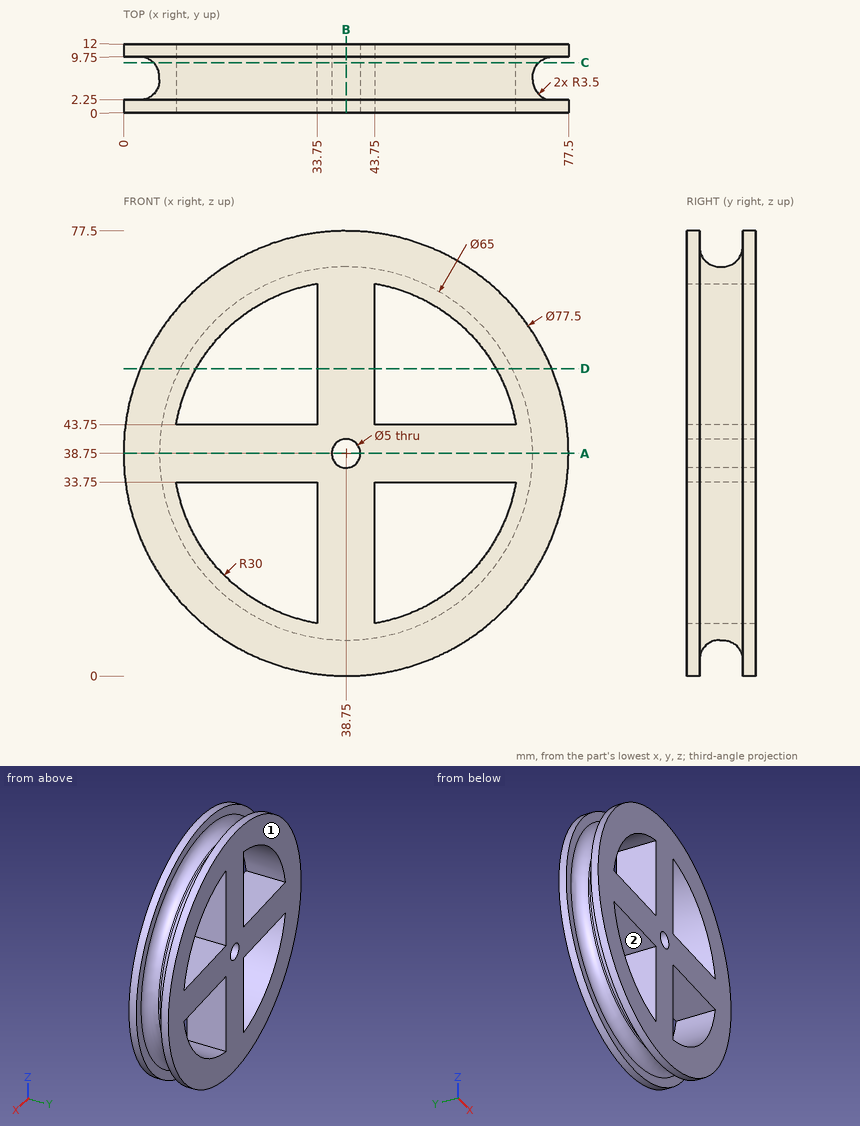
Verification items for this drawing (mm, ordinates from the low corner). A direction names the side the tool comes from. Round coordinates to 2 decimals unless told otherwise and drop trailing zeros. Order: outer loops, then holes, each group sorted by start corner. A loop starts at its lowest first (then second) coordinate and runs counter-clockwise, first axis right, second up. Notation, with made-up numbers: (31, 30.5) - (51, 30.5) arc R16 cw to (51, 60.5) - close; hole circle Ø5 at (64, 35). An arc over 180 degrees is marked (long way). Use CSV: the item, a comma, the result in double quotes.
(1) Section check C-C on y = 8.75. Record the boundary of the cut face in (x, z), and give its area (3 significant figures).
Entries:
outline,"circle Ø67.1 at (38.75, 38.75); hole (9.17, 33.75) arc R30 ccw to (33.75, 9.17) - (33.75, 33.75) - close; hole (9.17, 43.75) - (33.75, 43.75) - (33.75, 68.33) arc R30 ccw to start; hole circle Ø5 at (38.75, 38.75); hole (43.75, 9.17) arc R30 ccw to (68.33, 33.75) - (43.75, 33.75) - close; hole (43.75, 43.75) - (68.33, 43.75) arc R30 ccw to (43.75, 68.33) - close"
area,"1,780 mm^2"
(2) Access from +Z, -Z, +X, -X, +Y, -Y to the whole of each face (thin tool, end or side, straight path). Record for the marked faces 1 and 2.
Entries:
face 1,"+Z, -Z, +X, -X, +Y"
face 2,"+Y, -Y"
(3) Section check A-A on z = 38.75. Record the boundary of the cut face in (x, y).
Entries:
outline,"(0, 0) - (36.25, 0) - (36.25, 12) - (0, 12) - (0, 9.75) - (2.75, 9.75) arc R3.5 cw to (6.25, 6.25) - (6.25, 5.75) arc R3.5 cw to (2.75, 2.25) - (0, 2.25) - close; (41.25, 0) - (77.5, 0) - (77.5, 2.25) - (74.75, 2.25) arc R3.5 cw to (71.25, 5.75) - (71.25, 6.25) arc R3.5 cw to (74.75, 9.75) - (77.5, 9.75) - (77.5, 12) - (41.25, 12) - close"
(4) Section check B-B on x = 38.75. Record the boundary of the cut face in (y, z), and give its area (3 significant figures).
Entries:
outline,"(0, 0) - (2.25, 0) - (2.25, 2.75) arc R3.5 cw to (5.75, 6.25) - (6.25, 6.25) arc R3.5 cw to (9.75, 2.75) - (9.75, 0) - (12, 0) - (12, 36.25) - (0, 36.25) - close; (0, 41.25) - (12, 41.25) - (12, 77.5) - (9.75, 77.5) - (9.75, 74.75) arc R3.5 cw to (6.25, 71.25) - (5.75, 71.25) arc R3.5 cw to (2.25, 74.75) - (2.25, 77.5) - (0, 77.5) - close"
area,"787 mm^2"
(5) Section check D-D on z = 53.5. State how many separate pieces and enclosed holes the cut face has, and give its area (3 significant figures).
Entries:
separate pieces,"3"
enclosed holes,"0"
area,"262 mm^2"
(6) Gauge pin test, flat ends, axial feed: pin 1 Ø8 at (x, z) = (31.5, 8.5) entering from -Y; pin 2 Ø6 at (x, y) = (51.5, 9) entering from -Z; pin 3 Ø3 at (x, z) = (38.75, 38.75) entering from +Y; pin 4 Ø1 at (x, y) = (21.5, 5) entering from +Z. Record the tip position at first contact, or that the pin passes through.
Entries:
pin 1,"y = 0"
pin 2,"z = 1.27"
pin 3,"through"
pin 4,"z = 66.73"
(7) Thickness scan on probe 1 along X at (y, z) = (10.75, 23); probe 2 along X at (y, z) = (7.5, 44); probe 3 along Y at (x, z) = (71, 20). Record the ranges inside material, lowest first. Write a range as from..to.
Entries:
probe 1,"3.35..13.22, 33.75..43.75, 64.28..74.15"
probe 2,"6.44..9.21, 33.75..43.75, 68.29..71.06"
probe 3,"0..2.25, 9.75..12"
